```python
from build123d import *

# Parameters (mm, degrees)
SKETCH1_R           = 12.5
SKETCH1_R_2         = 8
BOSS_EXTRUDE1_DEPTH = 10
SKETCH3_R           = 1.5
CUT_EXTRUDE1_DEPTH  = 30.685855218
ESCALA1_SCALE       = 0.5


with BuildPart() as part:
    # Sketch1 → Boss-Extrude1 (new body)
    with BuildSketch(Plane(origin=(0, 0, 0), x_dir=(1, 0, 0), z_dir=(0, 1, 0))):
        with Locations(Location((0, 0, 0), (0, 0, 270))):
            Circle(SKETCH1_R)
        with Locations(Location((0, 0, 0), (0, 0, 270))):
            Circle(SKETCH1_R_2, mode=Mode.SUBTRACT)
    extrude(amount=BOSS_EXTRUDE1_DEPTH)

    # Sketch3 → Cut-Extrude1 (cut, through all)
    with BuildSketch(Plane.ZY.offset(12.5)):
        with Locations((0, 5)):
            Circle(SKETCH3_R)
    extrude(amount=-CUT_EXTRUDE1_DEPTH, mode=Mode.SUBTRACT)


with BuildPart() as part_1:
    # Escala1: scaled about (2.9522e-05, 5.000004154, -4.1694e-05)
    add(part.part.scale(ESCALA1_SCALE).moved(Location((1.4761e-05, 2.500002077, -2.0847e-05))))


solid = part_1.part
```
The model under review builds one solid part; all positions refer to its coordinate system, in mm. Round coordinates to 2 decimals unless told otherwise and drop trailing zeros. Order: outer loops, then holes, each group sorted by start corner. A loop starts at its lowest first (then second) coordinate and runs counter-clockwise, first axis right, second up.
Item 1: Add section C-C, the plane z = 2.5. State the section outline as (x, y) points.
Working result:
outline: (-5.73, 2.5) - (-3.12, 2.5) - (-3.12, 7.5) - (-5.73, 7.5) - close; (3.12, 2.5) - (5.73, 2.5) - (5.73, 7.5) - (3.12, 7.5) - close
Item 2: Draft analysis for pull direction Y (two halves, no side actions). For faces 1 (the flat face through (-4.1, 7.5, 1.3)), 2 (the cylindrical face through (5.073, 4.268, -0.163)), 3 (the flat face through (-4.1, 2.5, 1.3)), state which applies: released by +Y, released by -Y, zero draft, split by the parting line, or undercut.
Working result:
face 1: released by +Y
face 2: undercut
face 3: released by -Y
Item 3: Add section A-A, the plane x = 3. State the section outline as (y, z) points, and give its area (3 significant figures).
Working result:
outline: (2.5, -5.48) - (7.5, -5.48) - (7.5, -2.65) - (2.5, -2.65) - close; (2.5, 2.65) - (7.5, 2.65) - (7.5, 5.48) - (2.5, 5.48) - close
area: 28.4 mm2
Item 4: Add section B-B, the plane z = 0.25. State the section outline as (x, y) points, and give its area (3 significant figures).
Working result:
outline: (-6.24, 2.5) - (-3.99, 2.5) - (-3.99, 4.29) - (-6.24, 4.29) - close; (-6.24, 5.71) - (-3.99, 5.71) - (-3.99, 7.5) - (-6.24, 7.5) - close; (3.99, 2.5) - (6.25, 2.5) - (6.25, 4.29) - (3.99, 4.29) - close; (3.99, 5.71) - (6.25, 5.71) - (6.25, 7.5) - (3.99, 7.5) - close
area: 16.2 mm2
Item 5: Add section D-D, the plane x = -4.25. State the section outline as (y, z) points, and give its area (3 significant figures).
Working result:
outline: (2.5, -4.58) - (7.5, -4.58) - (7.5, 4.58) - (2.5, 4.58) - close; hole circle Ø1.5 at (5, 0)
area: 44.1 mm2
Item 6: To check wall thickness, follow probe 1 along X at (y, z) = (4.1, 0); probe 2 along Z at (x, y) = (-4, 4.9); probe 3 along Z at (x, y) = (2.25, 2.85). State the ranges of each line that lie inside material, in increasing order.
Working result:
probe 1: x = -6.25 to -4, 4 to 6.25
probe 2: z = -4.8 to -0.74, 0.74 to 4.8
probe 3: z = -5.83 to -3.31, 3.31 to 5.83
Item 7: For pin 1 (1.4 mm diameter, centred on y = 5, z = 0, fed in from +X); pin 2 (2 mm diameter, centred on x = -2.5, y = 6, fed in from -Z); pin 3 (3 mm diameter, centred on y = 5.5, z = 4, fed in from -X), all flat-tipped, find the tip position at first contact; note any pin that passes through.
Working result:
pin 1: passes through
pin 2: stops at z = -6.07
pin 3: stops at x = -5.73
